Geometry: final body of the model. Coordinates: model frame, mm. A direction names the side the tool comes from. Coordinates: 2 decimals unless noted, no trailing zeros. Order: outer loops, then holes, each group sorted by start corner. A loop starts at its lowest first (then second) coordinate and runs counter-clockwise, first axis right, second up. Notation, with made-up numbers: M 89,79.5 L 106,79.5 A10 ccw 106,85.5 Z; hole C 66.5,79.25 d7. An arc over 180 degrees is marked long. One line per question, with ' | ' between items.
from build123d import *

# Parameters (mm, degrees)
SKETCH1_W           = 101.6
SKETCH1_H           = 165.1
BOSS_EXTRUDE1_DEPTH = 50.8
SKETCH2_W           = 2.54
SKETCH2_H           = 2.54
CUT_EXTRUDE1_DEPTH  = 110.433918417
CHAMFER1_SIZE       = 10.16
SKETCH3_W           = 87.6
SKETCH3_H           = 143.876
CUT_EXTRUDE2_DEPTH  = 44.45
CUT_EXTRUDE3_DEPTH  = 2
SKETCH5_R           = 1.750000056
CUT_EXTRUDE4_DEPTH  = 110.433918417
SKETCH6_W           = 12.7
SKETCH6_H           = 6.999986
SKETCH6_H_2         = 6.999987499
CUT_EXTRUDE5_DEPTH  = 5.08
SKETCH7_W           = 15.494
SKETCH7_H           = 11.43
CUT_EXTRUDE6_DEPTH  = 110.433918417
SKETCH9_R           = 1.75
CUT_EXTRUDE7_DEPTH  = 5.08
SKETCH10_W          = 68.072
SKETCH10_H          = 19.558
BOSS_EXTRUDE2_DEPTH = 2.54
BOSS_EXTRUDE3_DEPTH = 25.4
SKETCH12_W          = 19.558
SKETCH12_H          = 41.91
CUT_EXTRUDE8_DEPTH  = 2.54


with BuildPart() as part:
    # Sketch1 → Boss-Extrude1 (new body)
    with BuildSketch(Plane(origin=(0, 0, 0), x_dir=(1, 0, 0), z_dir=(0, 1, 0))):
        Rectangle(SKETCH1_W, SKETCH1_H)
    extrude(amount=BOSS_EXTRUDE1_DEPTH)

    # Sketch2 → Cut-Extrude1 (cut, through all)
    with BuildSketch(Plane(origin=(0, 50.8, 0), x_dir=(1, 0, 0), z_dir=(0, 1, 0))):
        with Locations((-50.8, -63.5)):
            Rectangle(SKETCH2_W, SKETCH2_H)
        with Locations((50.8, -63.5)):
            Rectangle(SKETCH2_W, SKETCH2_H)
        with Locations((-50.8, -50.8)):
            Rectangle(SKETCH2_W, SKETCH2_H)
        with Locations((50.8, -50.8)):
            Rectangle(SKETCH2_W, SKETCH2_H)
        with Locations((-50.8, -38.1)):
            Rectangle(SKETCH2_W, SKETCH2_H)
        with Locations((50.8, -38.1)):
            Rectangle(SKETCH2_W, SKETCH2_H)
        with Locations((-50.8, -25.4)):
            Rectangle(SKETCH2_W, SKETCH2_H)
        with Locations((50.8, -25.4)):
            Rectangle(SKETCH2_W, SKETCH2_H)
        with Locations((-50.8, -12.7)):
            Rectangle(SKETCH2_W, SKETCH2_H)
        with Locations((50.8, -12.7)):
            Rectangle(SKETCH2_W, SKETCH2_H)
        with Locations((-50.8, 0)):
            Rectangle(SKETCH2_W, SKETCH2_H)
        with Locations((50.8, 0)):
            Rectangle(SKETCH2_W, SKETCH2_H)
        with Locations((-50.8, 12.7)):
            Rectangle(SKETCH2_W, SKETCH2_H)
        with Locations((50.8, 12.7)):
            Rectangle(SKETCH2_W, SKETCH2_H)
        with Locations((-50.8, 25.4)):
            Rectangle(SKETCH2_W, SKETCH2_H)
        with Locations((50.8, 25.4)):
            Rectangle(SKETCH2_W, SKETCH2_H)
        with Locations((-50.8, 38.1)):
            Rectangle(SKETCH2_W, SKETCH2_H)
        with Locations((50.8, 38.1)):
            Rectangle(SKETCH2_W, SKETCH2_H)
        with Locations((-50.8, 50.8)):
            Rectangle(SKETCH2_W, SKETCH2_H)
        with Locations((50.8, 50.8)):
            Rectangle(SKETCH2_W, SKETCH2_H)
        with Locations((-50.8, 63.5)):
            Rectangle(SKETCH2_W, SKETCH2_H)
        with Locations((50.8, 63.5)):
            Rectangle(SKETCH2_W, SKETCH2_H)
    extrude(amount=-CUT_EXTRUDE1_DEPTH, mode=Mode.SUBTRACT)

    # Chamfer1
    chamfer1_edges = [part.edges().sort_by_distance(p)[0] for p in [
        (50.8, 25.4, 82.55),
        (-50.8, 25.4, 82.55),
        (-50.8, 25.4, -82.55),
        (50.8, 25.4, -82.55),
    ]]
    chamfer(chamfer1_edges, length=CHAMFER1_SIZE)

    # Sketch3 → Cut-Extrude2 (cut)
    with BuildSketch(Plane(origin=(0, 50.8, 0), x_dir=(1, 0, 0), z_dir=(0, 1, 0))):
        with Locations((0, 3.612)):
            Rectangle(SKETCH3_W, SKETCH3_H)
    extrude(amount=-CUT_EXTRUDE2_DEPTH, mode=Mode.SUBTRACT)

    # Sketch4 → Cut-Extrude3 (cut)
    with BuildSketch(Plane(origin=(0, 50.8, 0), x_dir=(1, 0, 0), z_dir=(0, 1, 0))):
        Polygon((45.012893219, 76.762893219), (50.8, 70.975786438), (50.8, 72.39), (40.64, 82.55), (39.225786438, 82.55), align=None)
        Polygon((-45.012893219, -76.762893219), (-50.8, -70.975786438), (-50.8, -72.39), (-40.64, -82.55), (-39.225786438, -82.55), align=None)
    extrude(amount=-CUT_EXTRUDE3_DEPTH, mode=Mode.SUBTRACT)

    # Sketch5 → Cut-Extrude4 (cut, through all)
    with BuildSketch(Plane(origin=(0, 50.8, 0), x_dir=(1, 0, 0), z_dir=(0, 1, 0))):
        with Locations(Location((-25.4, -79.05, 0), (0, 0, 270))):
            Circle(SKETCH5_R)
        with Locations(Location((25.4, -79.05, 0), (0, 0, 270))):
            Circle(SKETCH5_R)
        with Locations(Location((25.4, 79.05, 0), (0, 0, 270))):
            Circle(SKETCH5_R)
        with Locations(Location((-25.4, 79.05, 0), (0, 0, 270))):
            Circle(SKETCH5_R)
    extrude(amount=-CUT_EXTRUDE4_DEPTH, mode=Mode.SUBTRACT)

    # Sketch6 → Cut-Extrude5 (cut)
    with BuildSketch(Plane.XZ):
        with Locations((-25.4, 79.050007)):
            Rectangle(SKETCH6_W, SKETCH6_H)
        with Locations((25.4, 79.050007)):
            Rectangle(SKETCH6_W, SKETCH6_H)
        with Locations((-25.4, -79.050007)):
            Rectangle(SKETCH6_W, SKETCH6_H)
        with Locations((25.4, -79.050006251)):
            Rectangle(SKETCH6_W, SKETCH6_H_2)
    extrude(amount=-CUT_EXTRUDE5_DEPTH, mode=Mode.SUBTRACT)

    # Sketch7 → Cut-Extrude6 (cut, through all)
    with BuildSketch(Plane.XZ):
        with Locations((0, 59.055)):
            Rectangle(SKETCH7_W, SKETCH7_H)
    extrude(amount=-CUT_EXTRUDE6_DEPTH, mode=Mode.SUBTRACT)

    # Sketch9 → Cut-Extrude7 (cut)
    with BuildSketch(Plane(origin=(0, 0, 68.326), x_dir=(-1, 0, 0), z_dir=(0, 0, -1))):
        with Locations((-9.933999944, 31.651)):
            Circle(SKETCH9_R)
        with Locations((10.187999944, 31.650999944)):
            Circle(SKETCH9_R)
        with Locations((10.187999944, 14.196)):
            Circle(SKETCH9_R)
        with Locations((-9.933999944, 14.069000056)):
            Circle(SKETCH9_R)
    extrude(amount=-CUT_EXTRUDE7_DEPTH, mode=Mode.SUBTRACT)

    # Sketch10 → Boss-Extrude2 (add)
    with BuildSketch(Plane(origin=(0, 6.35, 0), x_dir=(1, 0, 0), z_dir=(0, 1, 0))):
        with Locations((-9.764, -30.099)):
            Rectangle(SKETCH10_W, SKETCH10_H)
    extrude(amount=BOSS_EXTRUDE2_DEPTH)

    # Sketch11 → Boss-Extrude3 (add)
    with BuildSketch(Plane(origin=(0, 6.35, 0), x_dir=(1, 0, 0), z_dir=(0, 1, 0))):
        Polygon((-43.8, -43.688), (28.082, -43.688), (28.082, -20.32), (24.272, -20.32), (24.272, -39.878), (-43.8, -39.878), align=None)
    extrude(amount=BOSS_EXTRUDE3_DEPTH)

    # Sketch12 → Cut-Extrude8 (cut)
    with BuildSketch(Plane(origin=(-43.8, 0, 0), x_dir=(0, 0, -1), z_dir=(1, 0, 0))):
        with Locations((-30.099, 29.845)):
            Rectangle(SKETCH12_W, SKETCH12_H)
    extrude(amount=-CUT_EXTRUDE8_DEPTH, mode=Mode.SUBTRACT)


solid = part.part
1. Section B-B, the plane x = -25.4. Output: boundary loops of the cut face in (y, z), and give its area (3 significant figures).
Response values:
outline: M 0,-75.55 L 5.08,-75.55 L 5.08,-77.3 L 50.8,-77.3 L 50.8,-75.55 L 6.35,-75.55 L 6.35,20.32 L 8.89,20.32 L 8.89,39.88 L 31.75,39.88 L 31.75,43.69 L 6.35,43.69 L 6.35,68.33 L 50.8,68.33 L 50.8,77.3 L 5.08,77.3 L 5.08,75.55 L 0,75.55 Z; M 5.08,-82.55 L 50.8,-82.55 L 50.8,-80.8 L 5.08,-80.8 Z; M 5.08,80.8 L 50.8,80.8 L 50.8,82.55 L 5.08,82.55 Z | area: 1,750 mm^2
2. Section D-D, the plane y = 27. Give the number of separate pieces and of enclosed holes in the cut face, and give its area (3 significant figures).
Response values:
separate pieces: 1 | enclosed holes: 5 | area: 4,150 mm^2
3. Section A-A, the plane z = 59. Output: boundary loops of the cut face in (x, y).
Response values:
outline: M -50.8,0 L -7.75,0 L -7.75,6.35 L -43.8,6.35 L -43.8,50.8 L -50.8,50.8 Z; M 7.75,0 L 50.8,0 L 50.8,50.8 L 43.8,50.8 L 43.8,6.35 L 7.75,6.35 Z
4. Section C-C, the plane z = -79.05. Output: boundary loops of the cut face in (x, y).
Response values:
outline: M -44.14,0 L -31.75,0 L -31.75,5.08 L -27.15,5.08 L -27.15,50.8 L -44.14,50.8 Z; M -23.65,5.08 L -19.05,5.08 L -19.05,0 L 19.05,0 L 19.05,5.08 L 23.65,5.08 L 23.65,50.8 L -23.65,50.8 Z; M 27.15,5.08 L 31.75,5.08 L 31.75,0 L 44.14,0 L 44.14,48.8 L 42.73,48.8 L 42.73,50.8 L 27.15,50.8 Z
5. Material intervals for line 1 (Z direction, x = -10.5, y = 29.5); line 2 (X direction, y = 47, z = -8); line 3 (Z direction, x = 32.5, y = 17), sorted ascending. Write a range as [from, to].
Response values:
line 1: z = [-82.55, -75.55], [39.88, 43.69], [68.33, 82.55] | line 2: x = [-50.8, -43.8], [43.8, 50.8] | line 3: z = [-82.55, -75.55], [68.33, 82.55]
6. Draft query along Z for faces 1 (the face through (44.932, 49.814, -76.844)), 2 (the face through (-3, 31.75, 41)), 3 (the face through (45, 48.8, -77)). Return one class per face: pulls with the +Z half, pulls with the -Z half, needs draft (parallel to the pull), parting line crosses it, or undercut.
Response values:
face 1: pulls with the -Z half | face 2: undercut | face 3: needs draft
7. Pin query (flat end, axial travel): P1, Ø0.6, axis at x = -50.5, y = 16, coming from the +Z side; P2, Ø4.5, axis at x = -25.4, z = -79.05, coming from the -Y side; P3, Ø4, axis at x = 26.5, z = -12, coming from the +Y side. Return the tip coordinate at first contact, or that it passes through.
Response values:
P1: stops at z = 72.99 | P2: stops at y = 5.08 | P3: stops at y = 6.35
8. Access query for faces 4 (the face through (-50.8, 25, 6)), 5 (the face through (-45, 48.8, 77)), 6 (the face through (23.9, 5.08, 77.5)), 7 (the face through (24, 5.08, -81)), 8 (the face through (-8, 19, 43.688)). Directions: +Z, -Z, +X, -X, +Y, -Y. A direction counts if a zero-diameter tool reaches every point of the face in a straight line with its end or side. Return the directions, or none.
Response values:
face 4: +Z, -Z, -X, +Y, -Y | face 5: +Z, -X, +Y | face 6: +Z, -Y | face 7: -Z, -Y | face 8: +Y
